Source: CAD feature listing. Evaluate the final solid. Frame: model axes, mm. A direction names the side the tool comes from. Give positions to 0.01 mm unless a question says otherwise; leave off trailing zeros. Loops run counter-clockwise (first coordinate to the right, second up) from the corner with the lowest first, then second, coordinate; pieces in that order, holes last. Notation, with made-up numbers: M 89.5,71 L 93.5,71 A28 cw 93.5,94 Z; hole C -19.5,53 d1. An arc over 180 degrees is marked long. Answer in a Markdown table with one row per item.
```python
from build123d import *

# Parameters (mm, degrees)
SKETCH1_R           = 7.5
BOSS_EXTRUDE1_DEPTH = 3
FILLET1_R           = 1
CUT_EXTRUDE1_DEPTH  = 2
FILLET2_R           = 0.25


with BuildPart() as part:
    # Sketch1 → Boss-Extrude1 (new body)
    with BuildSketch(Plane(origin=(0, 0, 0), x_dir=(1, 0, 0), z_dir=(0, 1, 0))):
        with Locations(Location((0, 0, 0), (0, 0, 270))):  # turned: the seam where the file's is
            Circle(SKETCH1_R)
    extrude(amount=BOSS_EXTRUDE1_DEPTH)

    # Fillet1
    fillet1_edges = [part.edges().sort_by_distance(p)[0] for p in [
        (0, 0, -7.5),
    ]]
    fillet(fillet1_edges, radius=FILLET1_R)

    # Sketch2 → Cut-Extrude1 (cut)
    with BuildSketch(Plane.XZ):
        Polygon((-0.7, -0.7), (-0.7, -2.55), (0.7, -2.55), (0.7, -0.7), (2.55, -0.7), (2.55, 0.7), (0.7, 0.7), (0.7, 2.55), (-0.7, 2.55), (-0.7, 0.7), (-2.55, 0.7), (-2.55, -0.7), align=None)
    extrude(amount=-CUT_EXTRUDE1_DEPTH, mode=Mode.SUBTRACT)

    # Fillet2
    fillet2_edges = [part.edges().sort_by_distance(p)[0] for p in [
        (0.7, 0, -1.625),
        (1.625, 0, -0.7),
        (1.625, 0, 0.7),
        (0.7, 0, 1.625),
        (-0.7, 0, 1.625),
        (-1.625, 0, 0.7),
        (-1.625, 0, -0.7),
        (-0.7, 0, -1.625),
        (0, 3, -7.5),
    ]]
    fillet(fillet2_edges, radius=FILLET2_R)


solid = part.part
```
Q1. Section query A-A (y = 1.45). Output: boundary loops of the cut face in (x, z), plus the area to 3 significant figures.
Values follow:
| item | result |
|---|---|
| outline | C 0,0 d15; hole M -2.55,-0.7 L -0.7,-0.7 L -0.7,-2.55 L 0.7,-2.55 L 0.7,-0.7 L 2.55,-0.7 L 2.55,0.7 L 0.7,0.7 L 0.7,2.55 L -0.7,2.55 L -0.7,0.7 L -2.55,0.7 Z |
| area | 164 mm^2 |
Q2. Section query B-B (x = 0). Output: boundary loops of the cut face in (y, z).
Values follow:
| item | result |
|---|---|
| outline | M 0,-6.5 A1 ccw 1,-7.5 L 2.75,-7.5 A0.25 ccw 3,-7.25 L 3,7.25 A0.25 ccw 2.75,7.5 L 1,7.5 A1 ccw 0,6.5 L 0,2.55 L 2,2.55 L 2,-2.55 L 0,-2.55 Z |
Q3. Section query D-D (y = 2.35). Output: boundary loops of the cut face in (x, z).
Values follow:
| item | result |
|---|---|
| outline | C 0,0 d15 |
Q4. Ray query, probe 1 along X at (y, z) = (1.6, 0); probe 2 along Z at (x, y) = (0.75, 1.75); probe 3 along X at (y, z) = (1.8, -2.25). Return the intervals inside material, ascending. Write a range as from..to.
Values follow:
| item | result |
|---|---|
| probe 1 | -7.5..-2.55, 2.55..7.5 |
| probe 2 | -7.46..-0.7, 0.7..7.46 |
| probe 3 | -7.15..-0.7, 0.7..7.15 |
Q5. Section query C-C (z = 0). Output: boundary loops of the cut face in (x, y), plus the area to 3 significant figures.
Values follow:
| item | result |
|---|---|
| outline | M -7.5,1 A1 ccw -6.5,0 L -2.55,0 L -2.55,2 L 2.55,2 L 2.55,0 L 6.5,0 A1 ccw 7.5,1 L 7.5,2.75 A0.25 ccw 7.25,3 L -7.25,3 A0.25 ccw -7.5,2.75 Z |
| area | 34.3 mm^2 |
Q6. Mould query, pull axis Z, two halves, no side actions, for faces 1 (the cylindrical face through (0.33, 1.863, -7.493)), 2 (the flat face through (0, 3, 0)), 3 (the flat face through (0, 1, 2.55)). Classes: +Z half, -Z half, draft (parallel to the pull), parting line (faces both ways), or undercut.
Values follow:
| item | result |
|---|---|
| face 1 | parting line |
| face 2 | draft |
| face 3 | undercut |
Q7. Contact query for flat-ended pins moving along their axis: pin 1 Ø0.9 at (y, z) = (1.5, 2) entering from -X; pin 2 Ø0.5 at (x, y) = (-1.5, 1) entering from +Z; pin 3 Ø0.5 at (x, y) = (1.5, 1) entering from -Z; pin 4 Ø4 at (x, z) = (0.5, -1) entering from -Y. Output: stop coordinate, or through.
Values follow:
| item | result |
|---|---|
| pin 1 | x = -7.34 |
| pin 2 | z = 7.4 |
| pin 3 | z = -7.4 |
| pin 4 | y = 0 |
Q8. Reachability of faces 4 (the flat face through (-2, 1, 0.7)), 5 (the flat face through (-1.4, 0, 1.4)) from +Z, -Z, +X, -X, +Y, -Y: full face, straight path, thin tool, end or side. Return the list, or none.
Values follow:
| item | result |
|---|---|
| face 4 | -Y |
| face 5 | +Z, -Z, +X, -X, -Y |
